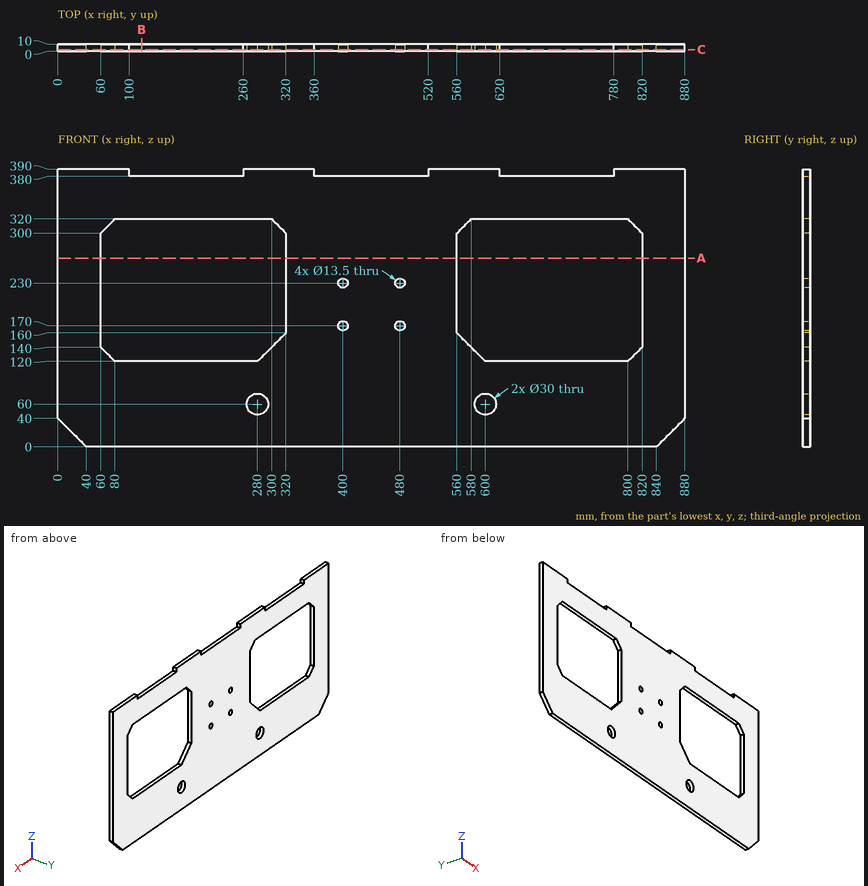
Design review of the part shown in the three views and the two pictorial views. Dimensions are in mm from the part's minimum x, y and z. Give positions to 0.01 mm unless a question says otherwise; leave off trailing zeros. Loops run counter-clockwise (first coordinate to the right, second up) from the corner with the lowest first, then second, coordinate; pieces in that order, holes last. Notation, with made-up numbers: M -37,11 L -9,11 A31 ccw -9,50 Z; hole C 44,-31 d3. An arc over 180 degrees is marked long. Answer as a JSON object with one key per item and string values. Group by question number.
Q1. Add section A-A on z = 265. Give the boundary of the cut face in (x, y).
Q2. Insertion check: P1, Ø2, axis at x = 605.5, y = 6, coming from the -Z side; P2, Ø8, axis at x = 400, z = 170, coming from the +Y side. Each pin has a flat end and moves straight along its axis. Give the tip position at first contact, or say it passes through.
Q3. Add section C-C on y = 2. Give the number of separate pieces and of enclosed holes in the cut face, and give its area (3 significant figures).
Q4. For probe 1 along X at (y, z) = (7.75, 170); probe 2 along X at (y, z) = (3.25, 209.5); probe 3 along Z at (x, y) = (400, 7.75), list the stretches that pass through material, from the lowest coordinate up. Write a range as [from, to].
Q5. Add section B-B on x = 117.5. Give the boundary of the cut face in (y, z), and give its area (3 significant figures).
Checked values:
{
 "1": {"outline": "M 0,0 L 60,0 L 60,10 L 0,10 Z; M 320,0 L 560,0 L 560,10 L 320,10 Z; M 820,0 L 880,0 L 880,10 L 820,10 Z"},
 "2": {"P1": "z = 0", "P2": "through"},
 "3": {"separate pieces": "1", "enclosed holes": "8", "area": "234,000 mm²"},
 "4": {"probe 1": "[0, 60], [320, 393.25], [406.75, 473.25], [486.75, 560], [820, 880]", "probe 2": "[0, 60], [320, 560], [820, 880]", "probe 3": "[0, 163.25], [176.75, 223.25], [236.75, 380]"},
 "5": {"outline": "M 0,0 L 10,0 L 10,120 L 0,120 Z; M 0,320 L 10,320 L 10,380 L 0,380 Z", "area": "1,800 mm²"}
}
